```python
from build123d import *

# Parameters (mm, degrees)
SKETCH1_R           = 7.5
BOSS_EXTRUDE1_DEPTH = 1.1
SKETCH2_R           = 6.5
BOSS_EXTRUDE2_DEPTH = 5
SKETCH3_R           = 3
CUT_EXTRUDE1_DEPTH  = 13.235603786
SKETCH4_R           = 6.5
SKETCH4_R_2         = 4
CUT_EXTRUDE2_DEPTH  = 0.08
CUT_EXTRUDE3_START  = -0.08
SKETCH5_R           = 5.5
SKETCH5_R_2         = 4
CUT_EXTRUDE3_DEPTH  = 0.08
FILLET1_R           = 0.31


with BuildPart() as part:
    # Sketch1 → Boss-Extrude1 (new body)
    with BuildSketch(Plane(origin=(0, 0, 0), x_dir=(1, 0, 0), z_dir=(0, 1, 0))):
        with Locations(Location((0, 0, 0), (0, 0, 270))):
            Circle(SKETCH1_R)
    extrude(amount=BOSS_EXTRUDE1_DEPTH)

    # Sketch2 → Boss-Extrude2 (add)
    with BuildSketch(Plane(origin=(0, 1.1, 0), x_dir=(1, 0, 0), z_dir=(0, 1, 0))):
        with Locations(Location((0, 0, 0), (0, 0, 270))):
            Circle(SKETCH2_R)
    extrude(amount=BOSS_EXTRUDE2_DEPTH)

    # Sketch3 → Cut-Extrude1 (cut, through all)
    with BuildSketch(Plane(origin=(0, 6.1, 0), x_dir=(1, 0, 0), z_dir=(0, 1, 0))):
        with Locations(Location((0, 0, 0), (0, 0, 270))):
            Circle(SKETCH3_R)
    extrude(amount=-CUT_EXTRUDE1_DEPTH, mode=Mode.SUBTRACT)

    # Sketch4 → Cut-Extrude2 (cut)
    with BuildSketch(Plane.XZ):
        with Locations(Location((0, 0, 0), (0, 0, 90))):
            Circle(SKETCH4_R)
        with Locations(Location((0, 0, 0), (0, 0, 270))):
            Circle(SKETCH4_R_2, mode=Mode.SUBTRACT)
    extrude(amount=-CUT_EXTRUDE2_DEPTH, mode=Mode.SUBTRACT)

    # Sketch5 → Cut-Extrude3 (cut)
    with BuildSketch(Plane(origin=(0, 6.1, 0), x_dir=(1, 0, 0), z_dir=(0, 1, 0)).offset(CUT_EXTRUDE3_START)):
        with Locations(Location((0, 0, 0), (0, 0, 270))):
            Circle(SKETCH5_R)
        with Locations(Location((0, 0, 0), (0, 0, 90))):
            Circle(SKETCH5_R_2, mode=Mode.SUBTRACT)
    extrude(amount=CUT_EXTRUDE3_DEPTH, mode=Mode.SUBTRACT)

    # Fillet1
    fillet1_edges = [part.edges().sort_by_distance(p)[0] for p in [
        (0, 0, -3),
        (0, 6.1, -3),
        (0, 0, -7.5),
        (0, 6.1, -6.5),
    ]]
    fillet(fillet1_edges, radius=FILLET1_R)


solid = part.part
```
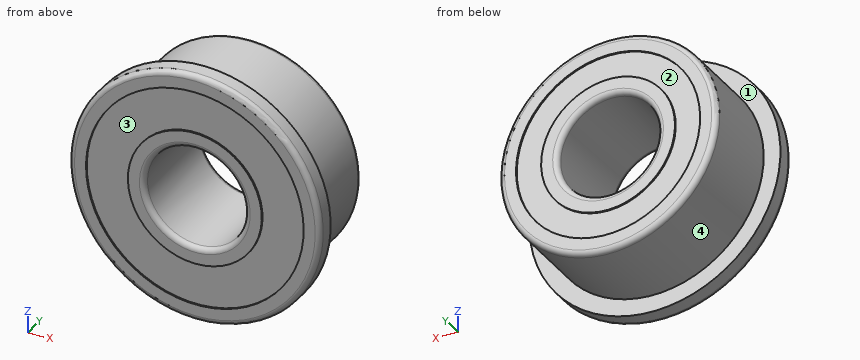
Could you check a few things on this model? Use its own coordinates, in mm. Face numbers are marked on the shaded views. Round coordinates to 2 decimals unless told otherwise and drop trailing zeros. Write each loop counter-clockwise with the first axis right and the second up, starting at its lowest first coordinate (ties: lowest second). Pieces come first, ordered by that corner, then holes.
(1) If I drill on probe 1 along X at (y, z) = (3.6, 0); probe 2 along Y at (x, z) = (-5.25, -2.5); probe 3 along Y at (x, z) = (3, 6.25), over which ranges is the centre line in solid material (lowest first)?
Findings below:
probe 1: x = -6.5 to -3, 3 to 6.5
probe 2: y = 0.08 to 6.1
probe 3: y = 0 to 1.1
(2) For pin 1 (5.5 mm diameter, centred on x = 0, z = 0, fed in from -Y); pin 2 (3 mm diameter, centred on x = -5.5, y = 4.5, fed in from +Z); pin 3 (1 mm diameter, centred on y = 2, z = 4, fed in from +X); pin 4 (2 mm diameter, centred on x = -5.5, y = 2.5, fed in from -Z), each with a flat end and sliding along its axis, tell me the tip position at first contact or that it passes through.
Findings below:
pin 1: passes through
pin 2: stops at z = 5.12
pin 3: stops at x = 5.48
pin 4: stops at z = -4.69
(3) Suppose I cut it at A-A on y = 2. Write out the boundary of the cut face in (x, z).
Findings below:
outline: circle Ø13 at (0, 0); hole circle Ø6 at (0, 0)
(4) Thinking about a two-plate mould opening in X: for the marked faces 1, 2, 3 and 4, which applies, +X half, -X half, draft (parallel to the pull), parting line (faces both ways), or undercut?
Findings below:
face 1: draft
face 2: undercut
face 3: undercut
face 4: parting line
